The model under review builds one solid part; all positions refer to its coordinate system, in mm. A direction names the side the tool comes from. Give positions to 0.01 mm unless a question says otherwise; leave off trailing zeros. Loops run counter-clockwise (first coordinate to the right, second up) from the corner with the lowest first, then second, coordinate; pieces in that order, holes last. Notation, with made-up numbers: M 37,-22 L 86,-22 A27 ccw 86,-3 Z; hole C 81,38 d6. An arc over 180 degrees is marked long. Return JSON: item names as keys, results as strings.
```python
from build123d import *

# Parameters (mm, degrees)
F1_DEPTH    = 19.05
F2_R        = 6.35
F0_W        = 19.05
F0_H        = 19.05
F3_DEPTH    = 7.62
F4_W        = 19.05
F4_H        = 7.62
F5_ANGLE    = 180
F6_T1_DEPTH = 39.37
F7_R        = 9.525
F8_DEPTH    = 19.051
F9_R        = 9.525
F10_DEPTH   = 12.7


# Not quite as in the source:
# - a fillet or chamfer that OpenCascade refuses, or shapes differently, is made with other operations: its cross-section is extruded or revolved along the edge and cut away or added


with BuildPart() as f1:
    # F0 (on Front) → F1 (new body)
    with BuildSketch(Plane.XZ):
        Polygon((50.8, -31.75), (50.8, 31.75), (-50.8, 31.75), (-50.8, -31.75), (-9.525, -31.75), (9.525, -31.75), align=None)
    extrude(amount=F1_DEPTH)

    # F2
    f2_edges = [f1.edges().sort_by_distance(p)[0] for p in [
        (50.8, -9.525, 31.75),
        (50.8, -9.525, -31.75),
        (-50.8, -9.525, -31.75),
        (-50.8, -9.525, 31.75),
    ]]
    fillet(f2_edges, radius=F2_R)

    # F0 (on Front) → F3 (join)
    with BuildSketch(Plane.XZ):
        with Locations((0, -41.275)):
            Rectangle(F0_W, F0_H)
    extrude(amount=F3_DEPTH)

    # F4 (on face) → F5 (revolve)
    with BuildSketch(Plane(origin=(0, 0, -50.8), x_dir=(1, 0, 0), z_dir=(0, 0, -1))):
        with Locations((0, 3.81)):
            Rectangle(F4_W, F4_H)
    revolve(axis=Axis((-4.1156476188, 30.4856614615, -50.8), (1, 0, 0)), revolution_arc=F5_ANGLE)

    # F6: fillet of radius 6.35 on 3 edges, made by hand

    # F6_s2 → F6_t1 (cut)
    with BuildSketch(Plane.XZ.offset(-84.4663229229)):
        with BuildLine():
            ThreePointArc((-9.525, -57.15), (-7.6651280605, -52.6598719395), (-3.175, -50.8))
            Line((-3.175, -50.8), (-9.525, -50.8))
            Line((-9.525, -50.8), (-9.525, -57.15))
        make_face()
        with BuildLine():
            ThreePointArc((9.525, -57.15), (7.6651280605, -52.6598719395), (3.175, -50.8))
            Line((3.175, -50.8), (9.525, -50.8))
            Line((9.525, -50.8), (9.525, -57.15))
        make_face()
    extrude(amount=F6_T1_DEPTH, mode=Mode.SUBTRACT)

    # F7 (on face) → F8 (cut, through all)
    with BuildSketch(Plane.XZ):
        with Locations((-25.4, 12.7)):
            Circle(F7_R)
        with Locations((25.4, 12.7)):
            Circle(F7_R)
    extrude(amount=F8_DEPTH, mode=Mode.SUBTRACT)

    # F9 (on face) → F10 (cut)
    with BuildSketch(Plane.XZ):
        with Locations((0, -6.35)):
            Circle(F9_R)
    extrude(amount=F10_DEPTH, mode=Mode.SUBTRACT)


solid = f1.part
```
1) Consider section D-D on z = -65. Write out the cut boundary in (x, y) (3 decimals).
From the geometry:
{"outline": "M -9.525,-4.875 L 9.525,-4.875 L 9.525,3.509 L -9.525,3.509 Z; M -9.525,57.462 L 9.525,57.462 L 9.525,65.847 L -9.525,65.847 Z"}
2) Consider section B-B on x = 25.4. Write out the cut boundary in (y, z) (3 decimals).
From the geometry:
{"outline": "M -19.05,-31.75 L 0,-31.75 L 0,3.175 L -19.05,3.175 Z; M -19.05,22.225 L 0,22.225 L 0,31.75 L -19.05,31.75 Z"}
3) Insertion check: pin 1 (9.5 mm diameter, centred on x = 4.5, z = -2.5, fed in from +Y); pin 2 (8 mm diameter, centred on x = 5.5, z = -71, fed in from -Y); pin 3 (7 mm diameter, centred on x = 0.5, y = 65.5, fed in from +Z). Each pin has a flat end and moves straight along its axis. Give the tip position at first contact, or say it passes through.
From the geometry:
{"pin 1": "y = 0", "pin 2": "y = -4", "pin 3": "z = -50.8"}
4) Consider section C-C on z = 12.7. Write out the cut boundary in (x, y) (3 decimals), then the cut area to 3 significant figures.
From the geometry:
{"outline": "M -50.8,-19.05 L -34.925,-19.05 L -34.925,0 L -50.8,0 Z; M -15.875,-19.05 L 15.875,-19.05 L 15.875,0 L -15.875,0 Z; M 34.925,-19.05 L 50.8,-19.05 L 50.8,0 L 34.925,0 Z", "area": "1,210 mm²"}
5) The part is to be moulded in two halves that separate along X. For faces 1 (the face through (7.714, 64.505, -52.71)), 2 (the face through (-2.06, -6.26, -15.65)), 3 (the face through (-27.46, -9.39, 3.4)), 4 (the face through (1, -9, 31.75)), say which applies: released by +X, released by -X, zero draft, split by the parting line, or undercut.
From the geometry:
{"face 1": "released by +X", "face 2": "undercut", "face 3": "undercut", "face 4": "zero draft"}
6) Tool access review of faces 5 (the face through (-12, 0, 0)), 6 (the face through (-9.525, 19, -80)), 7 (the face through (-7.714, 64.505, -52.71)): name each direction out of +Z, -Z, +X, -X, +Y, -Y from which nothing blocks a thin tool from reaching the whole face with its end or side.
From the geometry:
{"face 5": "+Z, +X, -X, +Y", "face 6": "-Z, -X, +Y, -Y", "face 7": "+Z, -X, +Y"}
7) Consider section A-A on y = -10. Write out the cut boundary in (x, z) (3 decimals), then the cut area to 3 significant figures.
From the geometry:
{"outline": "M -50.8,-25.4 A6.35 ccw -44.45,-31.75 L 44.45,-31.75 A6.35 ccw 50.8,-25.4 L 50.8,25.4 A6.35 ccw 44.45,31.75 L -44.45,31.75 A6.35 ccw -50.8,25.4 Z; hole C -25.4,12.7 d19.05; hole C 0,-6.35 d19.05; hole C 25.4,12.7 d19.05", "area": "5,560 mm²"}
8) Wall thickness on L1, parallel to X at y = -7, z = 12; L2, parallel to Z at x = 25.4, y = -10.5 (3 decimals); L3, parallel to Y at x = -24, z = -14: over which ranges is each line inside the solid? List them lowest first. Write a range as from..to.
From the geometry:
{"L1": "-50.8..-34.9, -15.9..15.9, 34.9..50.8", "L2": "-31.75..3.175, 22.225..31.75", "L3": "-19.05..0"}
